```python
from build123d import *

# Parameters (mm, degrees)
F0_W      = 20
F0_H      = 2
F2_T      = -0.5
F4_DEPTH  = 2
F6_DEPTH  = 25
F8_DEPTH  = 25
F10_DEPTH = 25
F12_DEPTH = 25


with BuildPart() as f1:
    # F0 (on Front) → F1 (revolve)
    with BuildSketch(Plane.XZ):
        with Locations((-10, 1)):
            Rectangle(F0_W, F0_H)
    revolve(axis=Axis((0, 0, 1), (0, 0, -1)))

    # F2
    f2_openings = [f1.faces().sort_by_distance(p)[0] for p in [
        (0, 0, 2),
    ]]
    offset(amount=F2_T, openings=f2_openings)

    # F3 (on Top) → F4 (join)
    with BuildSketch(Plane.XY):
        with BuildLine():
            Line((5, 20), (0, 20))
            ThreePointArc((0, 20), (2.520086, 19.840594), (5, 19.364917))
            Line((5, 19.364917), (5, 20))
        make_face()
        with BuildLine():
            ThreePointArc((19.364917, 5), (19.840594, 2.520086), (20, 0))
            Line((20, 0), (20, 5))
            Line((20, 5), (19.364917, 5))
        make_face()
        with BuildLine():
            Line((20, -5), (20, 0))
            ThreePointArc((20, 0), (19.840594, -2.520086), (19.364917, -5))
            Line((19.364917, -5), (20, -5))
        make_face()
        with BuildLine():
            ThreePointArc((5, -19.364917), (2.520086, -19.840594), (0, -20))
            Line((0, -20), (5, -20))
            Line((5, -20), (5, -19.364917))
        make_face()
        with BuildLine():
            Line((-5, -20), (0, -20))
            ThreePointArc((0, -20), (-2.520086, -19.840594), (-5, -19.364917))
            Line((-5, -19.364917), (-5, -20))
        make_face()
        with BuildLine():
            ThreePointArc((-19.364917, -5), (-19.840594, -2.520086), (-20, 0))
            Line((-20, 0), (-20, -5))
            Line((-20, -5), (-19.364917, -5))
        make_face()
        with BuildLine():
            Line((-20, 5), (-20, 0))
            ThreePointArc((-20, 0), (-19.840594, 2.520086), (-19.364917, 5))
            Line((-19.364917, 5), (-20, 5))
        make_face()
        with BuildLine():
            Line((0, 20), (-5, 20))
            Line((-5, 20), (-5, 19.364917))
            ThreePointArc((-5, 19.364917), (-2.520086, 19.840594), (0, 20))
        make_face()
    extrude(amount=F4_DEPTH)

    # F5 (on face) → F6 (join)
    with BuildSketch(Plane(origin=(0, 20, 0), x_dir=(-1, 0, 0), z_dir=(0, 1, 0))):
        Polygon((0, 1.333333), (-5, 0), (0, 0.666667), (5, 2), align=None)
    extrude(amount=F6_DEPTH)

    # F7 (on face) → F8 (join)
    with BuildSketch(Plane(origin=(-20, 0, 0), x_dir=(0, -1, 0), z_dir=(-1, 0, 0))):
        Polygon((0, 0.666667), (5, 2), (0, 1.333333), (-5, 0), align=None)
    extrude(amount=F8_DEPTH)

    # F9 (on face) → F10 (join)
    with BuildSketch(Plane.XZ.offset(20)):
        Polygon((0, 1.333333), (-5, 0), (0, 0.666667), align=None)
        Polygon((5, 2), (0, 1.333333), (0, 0.666667), align=None)
    extrude(amount=F10_DEPTH)

    # F11 (on face) → F12 (join)
    with BuildSketch(Plane.YZ.offset(20)):
        Polygon((0, 1.333333), (-5, 0), (0, 0.666667), align=None)
        Polygon((5, 2), (0, 1.333333), (0, 0.666667), align=None)
    extrude(amount=F12_DEPTH)


solid = f1.part
```
Read the model definition and answer for the solid it produces. Units are mm, in the model's axes. A direction names the side the tool comes from. Give positions to 0.01 mm unless a question says otherwise; leave off trailing zeros. Order: outer loops, then holes, each group sorted by start corner. A loop starts at its lowest first (then second) coordinate and runs counter-clockwise, first axis right, second up.
(1) Find section A-A (x = 11). Give the vertices of the cut face in (y, z).
(2) Find section B-B (y = 10). Give the vertices of the cut face in (x, z), plus the area to 3 significant figures.
(3) Given pin 1 (1.5 mm diameter, centred on x = 21, y = 8.5, fed in from -Z); pin 2 (0.5 mm diameter, centred on x = -20, z = 1, fed in from +Y); pin 3 (23.5 mm diameter, centred on x = 0, y = 0, fed in from +Z), each flat-ended and moving along its own axis, determine where each tip first touches the part or whether it passes through.
(4) Straight lines are drawn through the part: L1, parallel to X at y = 0, z = 1.55; L2, parallel to Y at x = 0, z = 1.25. For each, find the intervals that lie inside material, in ascending order.
(5) For faces 1 (the flat face through (2.465, 32.325, 0.676)), 2 (the flat face through (32.325, -2.465, 0.676)), 3 (the flat face through (-32.325, -2.465, 1.324)), 4 (the flat face through (20, 2, 1)), determine the directions among +Z, -Z, +X, -X, +Y, -Y from which every point of the face is accessible in a straight line to the end or side of a thin tool.
(6) Find section C-C (x = -36). Give the vertices of the cut face in (y, z).
Result sheet:
1. outline: (-16.7, 0) - (16.7, 0) - (16.7, 2) - (16.1, 2) - (16.1, 0.5) - (-16.1, 0.5) - (-16.1, 2) - (-16.7, 2) - close
2. outline: (-17.32, 0) - (17.32, 0) - (17.32, 2) - (16.74, 2) - (16.74, 0.5) - (-16.74, 0.5) - (-16.74, 2) - (-17.32, 2) - close
2. area: 19.1 mm2
3. pin 1: passes through
3. pin 2: stops at y = 5
3. pin 3: stops at z = 0.5
4. L1: x = -20 to -19.5, 19.5 to 20
4. L2: y = -45 to -19.5, 19.5 to 45
5. face 1: +Z, +X, +Y
5. face 2: +Z, +X, -Y
5. face 3: -Z, -X, -Y
5. face 4: -Z, +X, +Y
6. outline: (-5, 2) - (0, 0.67) - (5, 0) - (0, 1.33) - close
